Part model, mm, in its own coordinate system. A direction names the side the tool comes from. Give positions to 0.01 mm unless a question says otherwise; leave off trailing zeros. Loops run counter-clockwise (first coordinate to the right, second up) from the corner with the lowest first, then second, coordinate; pieces in that order, holes last. Notation, with made-up numbers: M 22.5,79 L 44.5,79 A26 cw 44.5,110 Z; hole C 9,35.25 d1. An arc over 180 degrees is marked long. Answer in a Markdown table with one row per item.
from build123d import *

# Parameters (mm, degrees)
BOSS_EXTRUDE1_DEPTH = 6.35
SKETCH2_R           = 1.7
CUT_EXTRUDE1_DEPTH  = 128.158650905
CUT_EXTRUDE2_DEPTH  = 128.158650905
BOSS_EXTRUDE2_DEPTH = 50.8


with BuildPart() as part:
    # Sketch1 → Boss-Extrude1 (new body)
    with BuildSketch(Plane(origin=(0, 0, 0), x_dir=(1, 0, 0), z_dir=(0, 1, 0))):
        Polygon((15.24, 53.34), (15.24, 66.04), (60.96, 66.04), (60.96, 0), (76.2, 0), (76.2, 101.6), (0, 101.6), (0, 0), (10, 0), (45.72, 0), (45.72, 53.34), align=None)
    extrude(amount=BOSS_EXTRUDE1_DEPTH)

    # Sketch2 → Cut-Extrude1 (cut, through all)
    with BuildSketch(Plane(origin=(0, 6.35, 0), x_dir=(1, 0, 0), z_dir=(0, 1, 0))):
        with Locations(Location((5, 96.6, 0), (0, 0, 270))):
            Circle(SKETCH2_R)
        with Locations(Location((71.2, 96.6, 0), (0, 0, 90))):
            Circle(SKETCH2_R)
        with Locations(Location((71.2, 5, 0), (0, 0, 270))):
            Circle(SKETCH2_R)
        with Locations(Location((5, 5, 0), (0, 0, 90))):
            Circle(SKETCH2_R)
    extrude(amount=-CUT_EXTRUDE1_DEPTH, mode=Mode.SUBTRACT)

    # Sketch3 → Cut-Extrude2 (cut, through all)
    with BuildSketch(Plane.ZY):
        Polygon((0, 3.175), (-20, 0), (0, 0), align=None)
    extrude(amount=-CUT_EXTRUDE2_DEPTH, mode=Mode.SUBTRACT)


with BuildPart() as body_2:
    # Mirror1: mirrored copy
    add(part.part.mirror(Plane.ZY.offset(25.4)))


with BuildPart() as part_1:
    add(part.part)

    add(body_2.part)  # Boss-Extrude2 merges body 2
    # Sketch4 → Boss-Extrude2 (add)
    with BuildSketch(Plane(origin=(-50.8, 0, 0), x_dir=(0, 0, -1), z_dir=(1, 0, 0))):
        Polygon((0, 6.35), (101.6, 6.35), (101.6, 0), (20, 0), (0, 3.175), align=None)
    extrude(amount=BOSS_EXTRUDE2_DEPTH)


solid = part_1.part
(1) Pull direction Z, two halves, no side cores. Call faces 1 (the face through (-89, 3, -66.04)), 2 (the face through (60.96, 3, -33)), 3 (the face through (-119.27, 1.61, -9.86)): +Z half, -Z half, draft (parallel to the pull), parting line (faces both ways), or undercut.
Recorded:
| item | result |
|---|---|
| face 1 | undercut |
| face 2 | draft |
| face 3 | +Z half |
(2) Saw through at D-D (z = -13.5). Write the cut outline in (x, y), plus the area to 3 significant figures.
Recorded:
| item | result |
|---|---|
| outline | M -127,1.03 L -111.76,1.03 L -111.76,6.35 L -127,6.35 Z; M -96.52,1.03 L 45.72,1.03 L 45.72,6.35 L -96.52,6.35 Z; M 60.96,1.03 L 76.2,1.03 L 76.2,6.35 L 60.96,6.35 Z |
| area | 919 mm^2 |
(3) Pin check, flat tips, straight feed: pin 1 Ø1.9 at (x, y) = (-99.5, 3.5) entering from +Z; pin 2 Ø5.5 at (x, z) = (-55.8, -5) entering from -Y. Stop position of each tip, or through.
Recorded:
| item | result |
|---|---|
| pin 1 | stops at z = -66.04 |
| pin 2 | stops at y = 1.94 |
(4) Which spindle directions (+Z, -Z, +X, -X, +Y, -Y) get a long thin tool onto all of the face, cutting with end or side? Do faces 4 (the face through (-96.52, 3, -26)), 5 (the face through (15.24, 3, -60)), 6 (the face through (-27, 0, -61)). Say none if no direction does.
Recorded:
| item | result |
|---|---|
| face 4 | +Z, +Y, -Y |
| face 5 | +Y, -Y |
| face 6 | +Z, -Z, +X, -X, -Y |
(5) Drill centre lines: line 1 along X through (y, z) = (3, -96.6); line 2 along X through (y, z) = (4.5, -12); line 3 along Z through (x, y) = (17, 4.5). Where is each one in solid material? Low to high.
Recorded:
| item | result |
|---|---|
| line 1 | x = -127 to -123.7, -120.3 to -57.5, -54.1 to 3.3, 6.7 to 69.5, 72.9 to 76.2 |
| line 2 | x = -127 to -111.76, -96.52 to 45.72, 60.96 to 76.2 |
| line 3 | z = -101.6 to -66.04, -53.34 to 0 |
(6) Saw through at B-B (z = -33). Write the cut outline in (x, y), plus the area to 3 significant figures.
Recorded:
| item | result |
|---|---|
| outline | M -127,0 L -111.76,0 L -111.76,6.35 L -127,6.35 Z; M -96.52,0 L 45.72,0 L 45.72,6.35 L -96.52,6.35 Z; M 60.96,0 L 76.2,0 L 76.2,6.35 L 60.96,6.35 Z |
| area | 1,100 mm^2 |
(7) Saw through at A-A (x = 32.5). Write the cut outline in (y, z) (3 decimals), plus the area to 3 significant figures.
Recorded:
| item | result |
|---|---|
| outline | M 0,-101.6 L 6.35,-101.6 L 6.35,-66.04 L 0,-66.04 Z; M 0,-53.34 L 6.35,-53.34 L 6.35,0 L 3.175,0 L 0,-20 Z |
| area | 533 mm^2 |
(8) Saw through at C-C (x = -13). Write the cut outline in (y, z) (3 decimals).
Recorded:
| item | result |
|---|---|
| outline | M 0,-101.6 L 6.35,-101.6 L 6.35,0 L 3.175,0 L 0,-20 Z |
